Could you check a few things on this model? Use its own coordinates, in mm. Coordinates: 2 decimals unless noted, no trailing zeros. Write each loop counter-clockwise with the first axis right and the second up, starting at its lowest first coordinate (ties: lowest second). Pieces come first, ordered by that corner, then holes. Notation, with made-up numbers: (32, 85) - (83, 85) arc R17 cw to (83, 98) - close; hole circle Ø6 at (65.5, 80.25). An arc over 180 degrees is marked (long way). Answer as a JSON object with one key per item and string values. Group by question number.
1) If we section it at A-A (x = 10.5): Write out the boundary of the cut face in (y, z).
2) We'd pull the mould along X, two halves only. Please class faces 1 (the cylindrical face through (1, -23, 25)), 2 (the flat face through (25, -12, 50)), 3 (the cylindrical face through (13.37, -12.68, 27.68)): released by +X, released by -X, zero draft, split by the parting line, or undercut.
3) If we section it at D-D (y = -23.5): Write out the boundary of the cut face in (x, z), plus the area to 3 significant figures.
4) If we section it at C-C (y = -16): Write out the boundary of the cut face in (x, z).
5) Will this pin go through, and if not, where does the flat tip stop? pin 1 Ø14 at (x, z) = (35.03, 18.67) entering from +Y.
6) Please list where these lines run through material, in increasing order: line 1 along Z through (x, y) = (15, -10); line 2 along X through (y, z) = (-21.25, 12.5); line 3 along Z through (x, y) = (40.5, -8.5).
7) If we section it at B-B (z = 35): Write out the boundary of the cut face in (x, y), plus the area to 3 significant figures.
```python
from build123d import *

# Parameters (mm, degrees)
F0_W     = 50
F0_H     = 50
F1_DEPTH = 25
F2_R     = 7.5
F3_DEPTH = 25
F4_R     = 5
F5_R     = 8.7642434369
F6_DEPTH = 25.001


with BuildPart() as f1:
    # F0 (on Front) → F1 (new body)
    with BuildSketch(Plane.XZ):
        with Locations((25, 25)):
            Rectangle(F0_W, F0_H)
    extrude(amount=F1_DEPTH)

    # F2 (on face) → F3 (cut)
    with BuildSketch(Plane.XZ.offset(25)):
        with Locations((15, 35)):
            Circle(F2_R)
    extrude(amount=-F3_DEPTH, mode=Mode.SUBTRACT)

    # F4
    f4_edges = [f1.edges().sort_by_distance(p)[0] for p in [
        (0, -12.5, 50),
        (0, -12.5, 0),
        (0, 0, 25),
        (0, -25, 25),
        (50, -12.5, 50),
        (25, 0, 50),
        (25, -25, 50),
        (50, -12.5, 0),
        (50, 0, 25),
        (50, -25, 25),
        (25, 0, 0),
        (25, -25, 0),
    ]]
    fillet(f4_edges, radius=F4_R)

    # F5 (on face) → F6 (cut, through all)
    with BuildSketch(Plane(origin=(0, 0, 0), x_dir=(-1, 0, 0), z_dir=(0, 1, 0))):
        with Locations((-35.0254848599, 18.6689179391)):
            Circle(F5_R)
    extrude(amount=-F6_DEPTH, mode=Mode.SUBTRACT)


solid = f1.part
```
Here are the results:
{
 "1": {"outline": "(-25, 5) arc R5 ccw to (-20, 0) - (-5, 0) arc R5 ccw to (0, 5) - (0, 29) - (-25, 29) - close; (-25, 41) - (0, 41) - (0, 45) arc R5 ccw to (-5, 50) - (-20, 50) arc R5 ccw to (-25, 45) - close"},
 "2": {"face 1": "released by -X", "face 2": "zero draft", "face 3": "undercut"},
 "3": {"outline": "(1.43, 5) arc R3.57 ccw to (5, 1.43) - (45, 1.43) arc R3.57 ccw to (48.57, 5) - (48.57, 45) arc R3.57 ccw to (45, 48.57) - (5, 48.57) arc R3.57 ccw to (1.43, 45) - close; hole circle Ø15 at (15, 35); hole circle Ø17.53 at (35.03, 18.67)", "area": "1,790 mm²"},
 "4": {"outline": "(0, 5) arc R5 ccw to (5, 0) - (45, 0) arc R5 ccw to (50, 5) - (50, 45) arc R5 ccw to (45, 50) - (5, 50) arc R5 ccw to (0, 45) - close; hole circle Ø15 at (15, 35); hole circle Ø17.53 at (35.03, 18.67)"},
 "5": {"pin 1": "passes through"},
 "6": {"line 1": "z = 0 to 27.5, 42.5 to 50", "line 2": "x = 0.16 to 28.8, 41.25 to 49.84", "line 3": "z = 0 to 11.82, 25.51 to 50"},
 "7": {"outline": "(0, -20) arc R5 ccw to (5, -25) - (7.5, -25) - (7.5, 0) - (5, 0) arc R5 ccw to (0, -5) - close; (22.5, -25) - (45, -25) arc R5 ccw to (50, -20) - (50, -5) arc R5 ccw to (45, 0) - (22.5, 0) - close", "area": "854 mm²"}
}
